Can you work these out from the model? Positions are in its coordinate system, mm. Face numbers are marked on the shaded views. Give positions to 0.01 mm unless a question says otherwise; leave off trailing zeros. Loops run counter-clockwise (first coordinate to the right, second up) from the corner with the lowest first, then second, coordinate; pieces in that order, holes last. Notation, with made-up numbers: (10, 65.5) - (42, 65.5) arc R12 cw to (42, 75.5) - close; hole circle Ø2 at (50, 5). An arc over 180 degrees is marked (long way). Answer in a Markdown table with one row per item.
from build123d import *

# Parameters (mm, degrees)
F3_START = -14
F2_R     = 3
F3_DEPTH = 10


with BuildPart() as f1:
    # F0 (on Front) → F1 (revolve)
    with BuildSketch(Plane.XZ):
        with BuildLine():
            Line((48.35, 0), (62.15, 0))
            Line((62.15, 0), (60.5, 21.2590787789))
            ThreePointArc((60.5, 21.2590787789), (59.9118794302, 22.5268121601), (58.6373248293, 23.1))
            Line((58.6373248293, 23.1), (48, 23.8))
            Line((48, 23.8), (48, 5.5))
            Line((48, 5.5), (48.35, 5.5))
            Line((48.35, 5.5), (48.35, 0))
        make_face()
    revolve(axis=Axis((0, 0, 11.9790900654), (0, 0, 1)))

    # F2 (on face) → F3 (cut)
    with BuildSketch(Plane(origin=(0, 0, 0), x_dir=(1, 0, 0), z_dir=(0, 0, -1)).offset(F3_START)):
        with Locations((-55, 0)):
            Circle(F2_R)
        with Locations((0, 55)):
            Circle(F2_R)
        with Locations((55, 0)):
            Circle(F2_R)
        with Locations((0, -55)):
            Circle(F2_R)
    extrude(amount=-F3_DEPTH, mode=Mode.SUBTRACT)


solid = f1.part
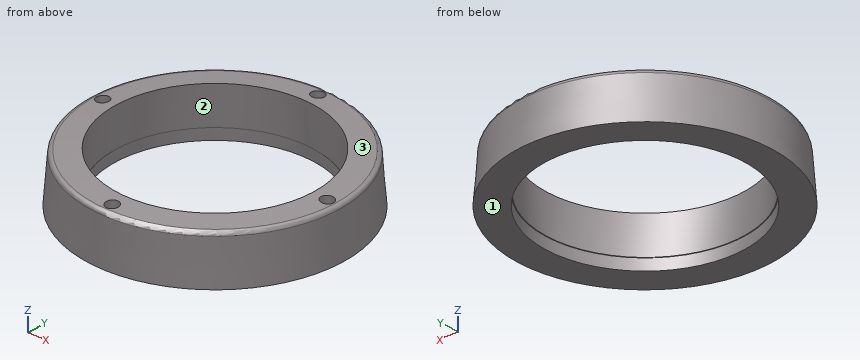
Q1. For pin 1 (1.8 mm diameter, centred on x = -54.5, y = -0.5, fed in from +Z); pin 2 (5 mm diameter, centred on x = 55.5, y = -1, fed in from +Z); pin 3 (1.5 mm diameter, centred on x = 41.5, y = 25, fed in from +Z); pin 4 (4 mm diameter, centred on y = -11, z = 3.5, fed in from +X), each with a flat end and sliding along its axis, tell me the tip position at first contact or that it passes through.
Checked values:
| item | result |
|---|---|
| pin 1 | stops at z = 14 |
| pin 2 | stops at z = 23.42 |
| pin 3 | stops at z = 23.8 |
| pin 4 | stops at x = 61.26 |
Q2. Imagine slicing it at C-C, the plane z = 9.25. Write out the boundary of the cut face in (x, y), and give its area (3 significant figures).
Checked values:
| item | result |
|---|---|
| outline | circle Ø122.86 at (0, 0); hole circle Ø96 at (0, 0) |
| area | 4,620 mm² |
Q3. If I drill on line 1 (Y direction, x = 0, z = 20.75); line 2 (X direction, y = -2, z = 6.5); line 3 (Y direction, x = 0, z = 3.7), over which ranges is the centre line in solid material (lowest first)? Write a range as [from, to].
Checked values:
| item | result |
|---|---|
| line 1 | y = [-60.54, -58], [-52, -48], [48, 52], [58, 60.54] |
| line 2 | x = [-61.61, -47.96], [47.96, 61.61] |
| line 3 | y = [-61.86, -48.35], [48.35, 61.86] |
Q4. Imagine slicing it at A-A, the plane y = 0. Write out the boundary of the cut face in (x, z), and give its area (3 significant figures).
Checked values:
| item | result |
|---|---|
| outline | (-62.15, 0) - (-48.35, 0) - (-48.35, 5.5) - (-48, 5.5) - (-48, 23.8) - (-52, 23.54) - (-52, 14) - (-58, 14) - (-58, 23.14) - (-58.64, 23.1) arc R2 ccw to (-60.5, 21.26) - close; (48, 5.5) - (48.35, 5.5) - (48.35, 0) - (62.15, 0) - (60.5, 21.26) arc R2 ccw to (58.64, 23.1) - (58, 23.14) - (58, 14) - (52, 14) - (52, 23.54) - (48, 23.8) - close |
| area | 502 mm² |
Q5. Imagine slicing it at B-B, the plane z = 19.25. Write out the boundary of the cut face in (x, y).
Checked values:
| item | result |
|---|---|
| outline | circle Ø121.31 at (0, 0); hole circle Ø6 at (-55, 0); hole circle Ø96 at (0, 0); hole circle Ø6 at (0, -55); hole circle Ø6 at (0, 55); hole circle Ø6 at (55, 0) |
Q6. If we mould it in two halves opening along Y, with no side actions, what happens to the marked faces 1, 2 and 3? For each: released by +Y, released by -Y, zero draft, split by the parting line, or undercut.
Checked values:
| item | result |
|---|---|
| face 1 | zero draft |
| face 2 | undercut |
| face 3 | split by the parting line |
